Geometry check sheet. Reference: the model listing, model coordinates, mm. A direction names the side the tool comes from. Give positions to 0.01 mm unless a question says otherwise; leave off trailing zeros. Loops run counter-clockwise (first coordinate to the right, second up) from the corner with the lowest first, then second, coordinate; pieces in that order, holes last. Notation, with made-up numbers: (4, 67) -> (29, 67) arc R20 cw to (29, 72) -> close; hole circle Ø3 at (20.25, -32). An arc over 180 degrees is marked (long way). Write each question's results on one line, items separated by ' | '. Start each with the question number.
1) Draft check along X on faces 1 (the face through (18.28, 4.27, -28.67)), 2 (the face through (28, 6.45, -18)), 3 (the face through (10.77, 1.67, 10.46)). Enter one of: pulls with the +X half, pulls with the -X half, needs draft (parallel to the pull), parting line crosses it, or undercut.
2) Sectioned sample at B-B on z = 0. Record the cut outline in (x, y), then the cut area to 3 significant figures.
3) Sectioned sample at D-D on y = 5. Record the cut outline in (x, z).
4) Set-up check for faces 4 (the face through (-31.476, 7.929, 9.912)), 5 (the face through (14.246, -3.689, -22.345)), 6 (the face through (0, 9.45, 0)): record each of +Z, -Z, +X, -X, +Y, -Y from which the full face is reachable in a straight line by a thin tool's end or side.
5) Sectioned sample at A-A on x = 0. Record the cut outline in (y, z).
6) Sectioned sample at C-C on y = -2.25. Record the cut outline in (x, z), then the cut area to 3 significant figures.
7) Depth check by flat-ended pin: pin 1 (6 mm diameter, centred on x = 1, y = -0.5, fed in from -Z); pin 2 (3 mm diameter, centred on x = -20.5, y = 2, fed in from -Z); pin 3 (2 mm diameter, centred on x = 10.61, z = -10.61, fed in from -Y). Enter the tip coordinate at first touch or a pass-through.
8) Scan lines: line 1 (Z direction, x = -11, y = -2.5); line 2 (Y direction, x = 31, z = 3.5); line 3 (X direction, y = 3.75, z = -1). Record each from-to range of solid material in increasing order. Write a range as from..to.
```python
from build123d import *

# Parameters (mm, degrees)
SKETCH3_R                 = 33
BOSS_EXTRUDE1_DEPTH       = 3
M3X0_5_TAPPED_HOLE1_D     = 2.5
M3X0_5_TAPPED_HOLE1_DEPTH = 7.5
M3X0_5_TAPPED_HOLE1_TIP   = 0.751075774


with BuildPart() as part:
    # Sketch2 → Revolve1 (revolve)
    with BuildSketch(Plane.XY):
        Polygon((0, -6.45), (0, 6.45), (34, 6.45), (34, 2.15), (26.5, -0.85), (26.5, -6.45), align=None)
    revolve(axis=Axis((0, -6.45, 0), (0, 1, 0)))

    # Sketch3 → Boss-Extrude1 (add)
    with BuildSketch(Plane(origin=(0, 6.45, 0), x_dir=(1, 0, 0), z_dir=(0, 1, 0))):
        with Locations(Location((0, 0, 0), (0, 0, 180))):
            Circle(SKETCH3_R)
    extrude(amount=BOSS_EXTRUDE1_DEPTH)

    # M3x0.5 Tapped Hole1
    with Locations(Plane(origin=(0, -6.45, 0), x_dir=(-1, 0, 0), z_dir=(0, -1, 0))):
        with Locations((10.606601718, -10.606601718), (-10.606601718, -10.606601718), (-10.606601718, 10.606601718), (10.606601718, 10.606601718)):
            Hole(M3X0_5_TAPPED_HOLE1_D / 2, depth=M3X0_5_TAPPED_HOLE1_DEPTH)
            with Locations((0, 0, -(M3X0_5_TAPPED_HOLE1_DEPTH + M3X0_5_TAPPED_HOLE1_TIP / 2))):  # 118° drill point
                Cone(0, M3X0_5_TAPPED_HOLE1_D / 2, M3X0_5_TAPPED_HOLE1_TIP, mode=Mode.SUBTRACT)


solid = part.part
```
Result:
1) face 1: parting line crosses it | face 2: needs draft | face 3: undercut
2) outline: (-34, 2.15) -> (-26.5, -0.85) -> (-26.5, -6.45) -> (26.5, -6.45) -> (26.5, -0.85) -> (34, 2.15) -> (34, 6.45) -> (33, 6.45) -> (33, 9.45) -> (-33, 9.45) -> (-33, 6.45) -> (-34, 6.45) -> close | area: 969 mm^2
3) outline: circle Ø68 at (0, 0)
4) face 4: +Y | face 5: -Y | face 6: +Z, -Z, +X, -X, +Y
5) outline: (-6.45, -26.5) -> (-0.85, -26.5) -> (2.15, -34) -> (6.45, -34) -> (6.45, -33) -> (9.45, -33) -> (9.45, 33) -> (6.45, 33) -> (6.45, 34) -> (2.15, 34) -> (-0.85, 26.5) -> (-6.45, 26.5) -> close
6) outline: circle Ø53 at (0, 0); hole circle Ø2.5 at (-10.61, -10.61); hole circle Ø2.5 at (-10.61, 10.61); hole circle Ø2.5 at (10.61, -10.61); hole circle Ø2.5 at (10.61, 10.61) | area: 2,190 mm^2
7) pin 1: z = -34 | pin 2: z = -28.19 | pin 3: y = 1.2
8) line 1: -24.11..-11.79, -9.42..9.42, 11.79..24.11 | line 2: 1.03..9.45 | line 3: -33.99..33.99
